Study the drawing (mm; zero at the part's minimum x, y, z) and answer. A direction names the side the tool comes from. Coordinates: 2 decimals unless noted, no trailing zeros. Loops run counter-clockwise (first coordinate to the right, second up) from the corner with the lowest first, then second, coordinate; pieces in that order, holes last. Notation, with made-up numbers: (-6.75, 60.25) -> (-1.75, 60.25) arc R19 ccw to (-1.75, 82.25) -> close; hole circle Ø10 at (79.5, 15.25). An arc over 180 degrees is marked (long way). Answer as CSV lines item,"result".
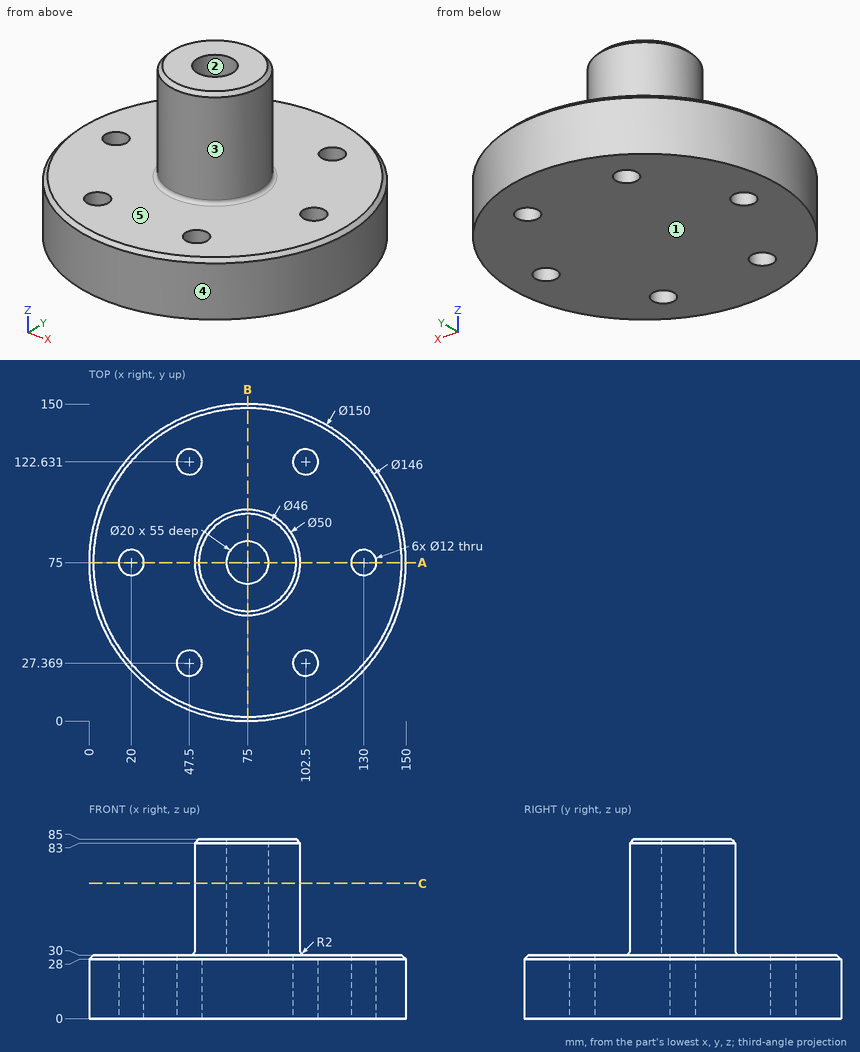
Q1. A cutting plane is placed at A-A, the plane y = 75. Write down the section's boundary in (x, z).
Results:
outline,"(0, 0) -> (14, 0) -> (14, 30) -> (2, 30) -> (0, 28) -> close; (26, 0) -> (124, 0) -> (124, 30) -> (102, 30) arc R2 cw to (100, 32) -> (100, 83) -> (98, 85) -> (85, 85) -> (85, 30) -> (65, 30) -> (65, 85) -> (52, 85) -> (50, 83) -> (50, 32) arc R2 cw to (48, 30) -> (26, 30) -> close; (136, 0) -> (150, 0) -> (150, 28) -> (148, 30) -> (136, 30) -> close"
Q2. A cutting plane is placed at B-B, the plane x = 75. Write down the section's boundary in (y, z), and give its area (3 significant figures).
Results:
outline,"(0, 0) -> (150, 0) -> (150, 28) -> (148, 30) -> (102, 30) arc R2 cw to (100, 32) -> (100, 83) -> (98, 85) -> (85, 85) -> (85, 30) -> (65, 30) -> (65, 85) -> (52, 85) -> (50, 83) -> (50, 32) arc R2 cw to (48, 30) -> (2, 30) -> (0, 28) -> close"
area,"6,140 mm²"
Q3. Find the intervals of material crossed by probe 1 along Y at (x, z) = (102.5, 13.25) (1 decimal); probe 2 along Y at (x, z) = (102, 19); probe 3 along Z at (x, y) = (70, 15.5), in increasing order. Write a range as [from, to].
Results:
probe 1,"y = [5.2, 21.4], [33.4, 116.6], [128.6, 144.8]"
probe 2,"y = [5.03, 21.39], [33.35, 116.65], [128.61, 144.97]"
probe 3,"z = [0, 30]"
Q4. Given pin 1 Ø4 at (x, z) = (88.5, 42) entering from -Y; pin 2 Ø12 at (x, z) = (95, 75) entering from +Y; pin 3 Ø6 at (y, z) = (70.5, 44.5) entering from +X (1 decimal), each flat-ended and moving along its own axis, determine where each tip first touches the part or whether it passes through.
Results:
pin 1,"stops at y = 52.8"
pin 2,"stops at y = 95.71"
pin 3,"stops at x = 100"
Q5. A cutting plane is placed at C-C, the plane z = 64. Write down the section's boundary in (x, y).
Results:
outline,"circle Ø50 at (75, 75); hole circle Ø20 at (75, 75)"
Q6. For the marked faces 4 and 5, determine the directions among +Z, -Z, +X, -X, +Y, -Y from which every point of the face is accessible in a straight line to the end or side of a thin tool.
Results:
face 4,"+Z, -Z"
face 5,"+Z"
Q7. For a pull along X with two mould halves and no side action, classify the marked faces 1, 2 and 3 as pulls with the +X half, pulls with the -X half, needs draft (parallel to the pull), parting line crosses it, or undercut.
Results:
face 1,"needs draft"
face 2,"undercut"
face 3,"parting line crosses it"
